```python
from build123d import *

# Parameters (mm, degrees)
SKETCH1_R                = 22.5
SKETCH1_R_2              = 15
BOSS_EXTRUDE1_DEPTH      = 30
BOSS_EXTRUDE1_DEPTH_BACK = 30
SKETCH2_R                = 3
CUT_EXTRUDE1_DEPTH       = 30


with BuildPart() as part:
    # Sketch1 → Boss-Extrude1 (new body, two sides)
    with BuildSketch(Plane.XY) as boss_extrude1_sk:
        Circle(SKETCH1_R)
        Circle(SKETCH1_R_2, mode=Mode.SUBTRACT)
    extrude(amount=BOSS_EXTRUDE1_DEPTH)
    extrude(boss_extrude1_sk.sketch, amount=-BOSS_EXTRUDE1_DEPTH_BACK)

    # Sketch2 → Cut-Extrude1 (cut)
    with BuildSketch(Plane(origin=(0, 0, 0), x_dir=(1, 0, 0), z_dir=(0, 1, 0))):
        with Locations((0, -15)):
            Circle(SKETCH2_R)
    cut_extrude1 = extrude(amount=CUT_EXTRUDE1_DEPTH, mode=Mode.SUBTRACT)

    # Mirror1: Cut-Extrude1 across plane
    add(cut_extrude1.mirror(Plane.XY), mode=Mode.SUBTRACT)


solid = part.part
```
Part model, mm, in its own coordinate system. A direction names the side the tool comes from. Round coordinates to 2 decimals unless told otherwise and drop trailing zeros. Write each loop counter-clockwise with the first axis right and the second up, starting at its lowest first coordinate (ties: lowest second). Pieces come first, ordered by that corner, then holes. Notation, with made-up numbers: (13.25, 44.5) -> (36.25, 44.5) arc R24 ccw to (36.25, 61.5) -> close; hole circle Ø5 at (12.25, 48). An arc over 180 degrees is marked (long way). Return JSON: item names as keys, results as strings. Group by question number.
Q1. Mould opens along X. For faces 3 (the cylindrical face through (-0.65, 18.55, 17.93)), 4 (the cylindrical face through (10.382, -19.961, 0.42)), 5 (the flat face through (15, -5, -30)) say: pulls with the +X half, pulls with the -X half, needs draft (parallel to the pull), parting line crosses it, or undercut.
Q2. Saw through at D-D on z = 23.5. Write the cut outline in (x, y), plus the area to 3 significant figures.
Q3. Saw through at A-A on x = 0. Write the cut outline in (y, z).
Q4. Saw through at C-C on x = -13. Write the cut outline in (y, z).
Q5. Which spindle directions (+Z, -Z, +X, -X, +Y, -Y) get a long thin tool onto all of the face, cutting with end or side? Do faces 1 (the flat face through (15, -5, 30)), 2 (the cylindrical face through (-0.65, 18.55, -17.93)). Say none if no direction does.
Q6. Saw through at B-B on y = 0. Write the cut outline in (x, z), plus the area to 3 significant figures.
Q7. Probe L1, parallel to Z at x = 0, y = 18; L2, parallel to Y at x = 0, z = 9; L3, parallel to Y at x = 0, z = 16. List the from-to ranges inside material, lowest first. Write a range as [from, to].
Q8. Pin check, flat tips, straight feed: pin 1 (6 mm diameter, centred on x = -16, z = -11.5, fed in from -Y); pin 2 (1 mm diameter, centred on y = 15.5, z = 8.5, fed in from +X); pin 3 (3 mm diameter, centred on x = -13, z = -22.5, fed in from -Y); pin 4 (18 mm diameter, centred on x = 0, y = 0, fed in from +Z). Stop position of each tip, or through.
Answer:
{
 "1": {"face 3": "undercut", "face 4": "parting line crosses it", "face 5": "needs draft"},
 "2": {"outline": "circle Ø45 at (0, 0); hole circle Ø30 at (0, 0)", "area": "884 mm2"},
 "3": {"outline": "(-22.5, -30) -> (-15, -30) -> (-15, 30) -> (-22.5, 30) -> close; (15, -30) -> (22.5, -30) -> (22.5, -18) -> (15, -18) -> close; (15, -12) -> (22.5, -12) -> (22.5, 12) -> (15, 12) -> close; (15, 18) -> (22.5, 18) -> (22.5, 30) -> (15, 30) -> close"},
 "4": {"outline": "(-18.36, -30) -> (-7.48, -30) -> (-7.48, 30) -> (-18.36, 30) -> close; (7.48, -30) -> (18.36, -30) -> (18.36, 30) -> (7.48, 30) -> close"},
 "5": {"face 1": "+Z, +X, -X, +Y, -Y", "face 2": "+Y"},
 "6": {"outline": "(-22.5, -30) -> (-15, -30) -> (-15, 30) -> (-22.5, 30) -> close; (15, -30) -> (22.5, -30) -> (22.5, 30) -> (15, 30) -> close", "area": "900 mm2"},
 "7": {"L1": "[-30, -18], [-12, 12], [18, 30]", "L2": "[-22.5, -15], [15, 22.5]", "L3": "[-22.5, -15]"},
 "8": {"pin 1": "y = -18.36", "pin 2": "x = 16.77", "pin 3": "y = -19.34", "pin 4": "through"}
}
